```python
from build123d import *

# Parameters (mm, degrees)
SKETCH1_W                = 6
SKETCH1_H                = 1.2
SKETCH1_W_2              = 1.2
SKETCH1_H_2              = 4.3
REVOLVE1_ANGLE           = 180
REVOLVE2_START           = 4.3
REVOLVE2_DEPTH           = 2.7
SKETCH3_W                = 6.5
SKETCH3_H                = 1.5
CUT_EXTRUDE1_DEPTH       = 10
CUT_EXTRUDE2_DEPTH       = 10
SKETCH5_W                = 2
SKETCH5_H                = 2
BOSS_EXTRUDE1_DEPTH      = 1.2
SKETCH6_W                = 1.2
SKETCH6_H                = 3
BOSS_EXTRUDE2_DEPTH      = 1.5
CHAMFER1_SIZE            = 0.5
CHAMFER1_OF_MIRROR1_SIZE = 0.5
SKETCH7_W                = 2.9
SKETCH7_H                = 1.2
BOSS_EXTRUDE3_DEPTH      = 5
BOSS_EXTRUDE4_DEPTH      = 0.6
FILLET1_R                = 0.5


# Read off the part's stored shape, not the designer's step: Revolve2
with BuildPart() as part:
    # Sketch1 → Revolve1 (revolve)
    with BuildSketch(Plane.XY):
        with Locations((3, -0.6)):
            Rectangle(SKETCH1_W, SKETCH1_H)
        with Locations((6.6, -0.6)):
            Rectangle(SKETCH1_W_2, SKETCH1_H)
        with Locations((6.6, 2.15)):
            Rectangle(SKETCH1_W_2, SKETCH1_H_2)
    revolve(axis=Axis((0, -1.2, 0), (0, 1, 0)), revolution_arc=REVOLVE1_ANGLE)

    # Revolve2 outline → Revolve2 (add)
    with BuildSketch(Plane(origin=(0, 0, 0), x_dir=(1, 0, 0), z_dir=(0, 1, 0)).offset(REVOLVE2_START)):
        with BuildLine():
            ThreePointArc((3.7, 6.176568627), (0, 7.2), (-3.7, 6.176568627))
            Line((-3.7, 6.176568627), (-3.7, 4.723346271))
            ThreePointArc((-3.7, 4.723346271), (0, 6), (3.7, 4.723346271))
            Line((3.7, 4.723346271), (3.7, 6.176568627))
        make_face()
    extrude(amount=REVOLVE2_DEPTH)

    # Sketch3 → Cut-Extrude1 (cut)
    with BuildSketch(Plane.XY):
        with Locations((0, 0.75)):
            Rectangle(SKETCH3_W, SKETCH3_H)
    extrude(amount=-CUT_EXTRUDE1_DEPTH, mode=Mode.SUBTRACT)

    # Sketch4 → Cut-Extrude2 (cut)
    with BuildSketch(Plane(origin=(0, 0, 0), x_dir=(1, 0, 0), z_dir=(0, 1, 0))):
        Polygon((-1.45, 3.3), (-3.6, 3.3), (-3.6, 0), (3.6, 0), (3.6, 3.3), (1.45, 3.3), (1.45, 0.8), (-1.45, 0.8), align=None)
    extrude(amount=-CUT_EXTRUDE2_DEPTH, mode=Mode.SUBTRACT)

    # Sketch5 → Boss-Extrude1 (add)
    with BuildSketch(Plane(origin=(0, 0, 0), x_dir=(1, 0, 0), z_dir=(0, 1, 0))):
        with Locations((-4.6, -1)):
            Rectangle(SKETCH5_W, SKETCH5_H)
        with Locations((4.6, -1)):
            Rectangle(SKETCH5_W, SKETCH5_H)
    extrude(amount=-BOSS_EXTRUDE1_DEPTH)

    # Sketch6 → Boss-Extrude2 (add)
    with BuildSketch(Plane(origin=(6, 0, 0), x_dir=(0, 0, -1), z_dir=(1, 0, 0))):
        with Locations((-0.6, 1.55)):
            Rectangle(SKETCH6_W, SKETCH6_H)
    boss_extrude2 = extrude(amount=BOSS_EXTRUDE2_DEPTH)

    # Chamfer1
    chamfer1_edges = [part.edges().sort_by_distance(p)[0] for p in [
        (7.5, 1.55, 1.2),
    ]]
    chamfer(chamfer1_edges, length=CHAMFER1_SIZE)

    # Mirror1: Boss-Extrude2 across plane
    add(boss_extrude2.mirror(Plane(origin=(0, 0, 0), x_dir=(0, 0, 1), z_dir=(1, 0, 0))))

    # Chamfer1 of Mirror1
    chamfer1_of_mirror1_edges = [part.edges().sort_by_distance(p)[0] for p in [
        (-7.5, 1.55, 1.2),
    ]]
    chamfer(chamfer1_of_mirror1_edges, length=CHAMFER1_OF_MIRROR1_SIZE)

    # Sketch7 → Boss-Extrude3 (add)
    with BuildSketch(Plane.XZ.offset(1.2)):
        with Locations((0, -1.4)):
            Rectangle(SKETCH7_W, SKETCH7_H)
    extrude(amount=BOSS_EXTRUDE3_DEPTH)

    # Sketch8 → Boss-Extrude4 (add, symmetric)
    with BuildSketch(Plane(origin=(0, 0, 0), x_dir=(0, 0, -1), z_dir=(1, 0, 0))):
        Polygon((2, -6.2), (6, -1.2), (2, -1.2), align=None)
    extrude(amount=BOSS_EXTRUDE4_DEPTH, both=True)

    # Fillet1
    fillet1_edges = [part.edges().sort_by_distance(p)[0] for p in [
        (-1.45, -6.2, -1.4),
        (1.45, -6.2, -1.4),
    ]]
    fillet(fillet1_edges, radius=FILLET1_R)


solid = part.part
```
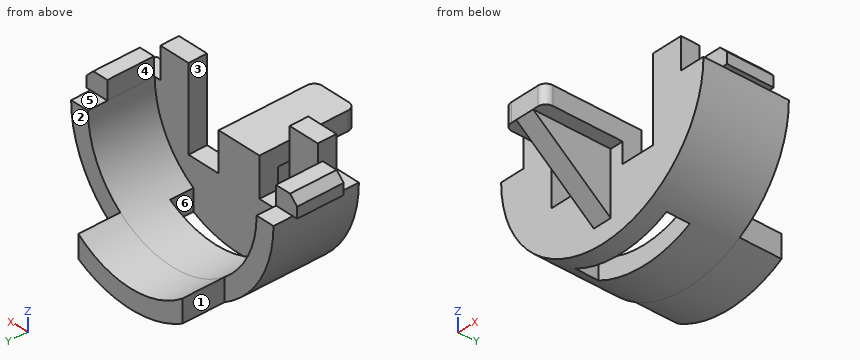
CAD build for the part. Positions are in the model's coordinates, mm. Face numbers are marked on the shaded views. A direction names the side the tool comes from. Round coordinates to 2 decimals unless told otherwise and drop trailing zeros. Loops run counter-clockwise (first coordinate to the right, second up) from the corner with the lowest first, then second, coordinate; pieces in that order, holes last. Notation, with made-up numbers: M 54,-7 L 80,-7 A30 ccw 80,32 Z; hole C 70,-28 d1. An arc over 180 degrees is marked long. Use a Markdown table: item, result. Add a question column.
(1) Cut at D-D (z = -1.5). Give the cut face in (x, y), and give its area (3 significant figures).
(2) Flat gauge pins, fed straight in: pin 1 (3 mm diameter, centred on x = 1, z = -1, fed in from +Y); pin 2 (1.3 mm diameter, centred on x = -7, z = 1, fed in from +Y); pin 3 (3 mm diameter, centred on x = -1, y = -1, fed in from +Z); pin 4 (5 mm diameter, centred on y = 3.5, z = -2, fed in from +X). Where does each tip first touch, or does it go through?
(3) Drill centre lines: line 1 (Y direction, x = -2.25, z = -5); line 2 (X direction, y = 0.75, z = -5.25); line 3 (X direction, y = 3, z = -0.5). Where is each one in solid material? Low to high.
(4) Pull direction X, two halves, no side cores. Call the marked faces 1, 2 and 3: +X half, -X half, draft (parallel to the pull), parting line (faces both ways), or undercut.
(5) Which spindle directions (+Z, -Z, +X, -X, +Y, -Y) get a long thin tool onto all of the face, cutting with end or side? Do the marked faces 4, 5 and 6. Say none if no direction does.
(6) Cut at B-B (x = 0). Give the cut face in (y, z), and give its area (3 significant figures).
(7) Cut at C-C (z = 0.5). Give the cut face in (x, y), and give its area (3 significant figures).
(8) Cut at A-A (y = 0.25). Give the cut face in (x, z), and give its area (3 significant figures).
Geometry says:
| question | item | result |
|---|---|---|
| 1 | outline | M -7.04,-1.2 L -3.6,-1.2 L -3.6,0 L -5.81,0 L -5.81,4.3 L -7.04,4.3 Z; M -1.45,-5.7 A0.5 ccw -0.95,-6.2 L 0.95,-6.2 A0.5 ccw 1.45,-5.7 L 1.45,0 L -1.45,0 Z; M 3.6,-1.2 L 7.04,-1.2 L 7.04,4.3 L 5.81,4.3 L 5.81,0 L 3.6,0 Z |
| 1 | area | 36.7 mm² |
| 2 | pin 1 | stops at y = 0 |
| 2 | pin 2 | stops at y = 3.05 |
| 2 | pin 3 | stops at z = -0.8 |
| 2 | pin 4 | stops at x = 7.5 |
| 3 | line 1 | y = -1.2 to 0 |
| 3 | line 2 | x = -4.93 to -3.25, 3.25 to 4.93 |
| 3 | line 3 | x = -7.18 to -5.98, 5.98 to 7.18 |
| 4 | face 1 | -X half |
| 4 | face 2 | draft |
| 4 | face 3 | undercut |
| 5 | face 4 | +Z, +Y, -Y |
| 5 | face 5 | +Z, +X, -X, +Y |
| 5 | face 6 | +Z, -Z |
| 6 | outline | M -6.2,-2 L -1.2,-6 L -1.2,-7.2 L 0,-7.2 L 0,-0.8 L -6.2,-0.8 Z; M 1.5,-7.2 L 7,-7.2 L 7,-6 L 1.5,-6 Z |
| 6 | area | 30.3 mm² |
| 7 | outline | M -7.5,0.05 L -6,0.05 L -6,3.05 L -7.5,3.05 Z; M -5.6,-1.2 L -3.6,-1.2 L -3.6,0 L -5.6,0 Z; M 3.6,-1.2 L 5.6,-1.2 L 5.6,0 L 3.6,0 Z; M 6,0.05 L 7.5,0.05 L 7.5,3.05 L 6,3.05 Z |
| 7 | area | 13.8 mm² |
| 8 | outline | M -7.5,0 L -7.2,0 A7.2 ccw -3.25,-6.42 L -3.25,-5.04 A6 cw -6,0 L -6,1.2 L -7,1.2 L -7.5,0.7 Z; M 3.25,-6.42 A7.2 ccw 7.2,0 L 7.5,0 L 7.5,0.7 L 7,1.2 L 6,1.2 L 6,0 A6 cw 3.25,-5.04 Z |
| 8 | area | 20.1 mm² |
